For this review, use the dimensioned drawing (mm, ordinates from the lowest corner) and the shaded views. A direction names the side the tool comes from. Give positions to 0.01 mm unless a question says otherwise; leave off trailing zeros. Order: outer loops, then holes, each group sorted by start corner. A loop starts at its lowest first (then second) coordinate and runs counter-clockwise, first axis right, second up.
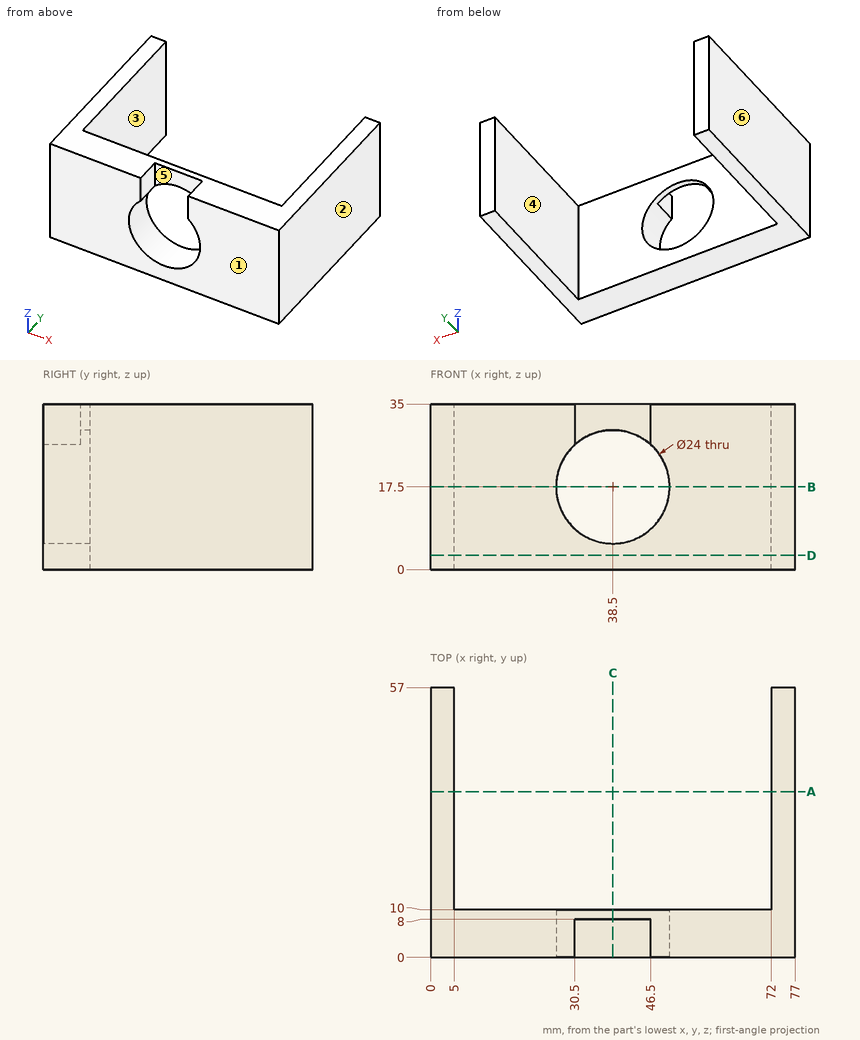
1. Draft analysis for pull direction X (two halves, no side actions). For the marked faces 1, 2 and 3, state which applies: pulls with the +X half, pulls with the -X half, needs draft (parallel to the pull), parting line crosses it, or undercut.
Recorded:
face 1: needs draft
face 2: pulls with the +X half
face 3: undercut
2. Take a section at B-B (z = 17.5). State the section outline as (x, y) points.
Recorded:
outline: (0, 0) - (26.5, 0) - (26.5, 10) - (5, 10) - (5, 57) - (0, 57) - close; (50.5, 0) - (77, 0) - (77, 57) - (72, 57) - (72, 10) - (50.5, 10) - close
3. Take a section at C-C (x = 38.5). State the section outline as (y, z) points, then the cut area to 3 significant figures.
Recorded:
outline: (0, 0) - (10, 0) - (10, 5.5) - (0, 5.5) - close; (8, 29.5) - (10, 29.5) - (10, 35) - (8, 35) - close
area: 66.0 mm2
4. Take a section at A-A (y = 35). State the section outline as (x, z) points.
Recorded:
outline: (0, 0) - (5, 0) - (5, 35) - (0, 35) - close; (72, 0) - (77, 0) - (77, 35) - (72, 35) - close
5. Machinability: for the marked faces 4, 5 and 6, which of the approach directions +Z, -Z, +X, -X, +Y, -Y give a long, thin tool a straight path to every point of the face, cutting with its end or side? Answer none if there is none.
Recorded:
face 4: +Z, -Z, +Y
face 5: +Z, -Y
face 6: +Z, -Z, -X, +Y, -Y
6. Take a section at D-D (z = 3). State the section outline as (x, y) points.
Recorded:
outline: (0, 0) - (77, 0) - (77, 57) - (72, 57) - (72, 10) - (5, 10) - (5, 57) - (0, 57) - close
7. For pin 1 (4.5 mm diameter, centred on x = 41, z = 29, fed in from -Y); pin 2 (19 mm diameter, centred on x = 38.5, z = 17.5, fed in from +Y); pin 3 (12 mm diameter, centred on x = 65, z = 8, fed in from +Y), all flat-tipped, find the tip position at first contact; note any pin that passes through.
Recorded:
pin 1: stops at y = 8
pin 2: passes through
pin 3: stops at y = 10
8. For line 1 along X through (y, z) = (24.5, 30.5); line 2 along X through (y, z) = (5.25, 17.5); line 3 along Y through (x, z) = (25.5, 25), list the stretches that pass through material, from the lowest coordinate up.
Recorded:
line 1: x = 0 to 5, 72 to 77
line 2: x = 0 to 26.5, 50.5 to 77
line 3: y = 0 to 10
